```python
from build123d import *

# Parameters (mm, degrees)
SKETCH1_R           = 6.9
BOSS_EXTRUDE1_DEPTH = 24.8
SKETCH2_R           = 1.9
CUT_EXTRUDE1_DEPTH  = 24.8
SKETCH3_R           = 4
CUT_EXTRUDE2_DEPTH  = 10
SKETCH4_R           = 2
CUT_EXTRUDE3_DEPTH  = 10


with BuildPart() as part:
    # Sketch1 → Boss-Extrude1 (new body)
    with BuildSketch(Plane.XY):
        with Locations(Location((0.333575811, 0, 0), (0, 0, 180))):
            Circle(SKETCH1_R)
    extrude(amount=BOSS_EXTRUDE1_DEPTH)

    # Sketch2 → Cut-Extrude1 (cut)
    with BuildSketch(Plane(origin=(0, 6.9, 0), x_dir=(1, 0, 0), z_dir=(0, 1, 0))):
        with Locations(Location((0.515412316, -4, 0), (0, 0, 270))):
            Circle(SKETCH2_R)
        with Locations(Location((0.515412316, -20.8, 0), (0, 0, 270))):
            Circle(SKETCH2_R)
    extrude(amount=-CUT_EXTRUDE1_DEPTH, mode=Mode.SUBTRACT)

    # Sketch3 → Cut-Extrude2 (cut)
    with BuildSketch(Plane.XY.offset(24.8)):
        Circle(SKETCH3_R)
    extrude(amount=-CUT_EXTRUDE2_DEPTH, mode=Mode.SUBTRACT)

    # Sketch4 → Cut-Extrude3 (cut)
    with BuildSketch(Plane(origin=(0, 0, 0), x_dir=(-1, 0, 0), z_dir=(0, 0, -1))):
        Circle(SKETCH4_R)
    extrude(amount=-CUT_EXTRUDE3_DEPTH, mode=Mode.SUBTRACT)


solid = part.part
```
Design review of the part built by this model. Coordinates are the model's own, in mm. A direction names the side the tool comes from. Give positions to 0.01 mm unless a question says otherwise; leave off trailing zeros. Write each loop counter-clockwise with the first axis right and the second up, starting at its lowest first coordinate (ties: lowest second). Pieces come first, ordered by that corner, then holes. Notation, with made-up numbers: (65.5, -25) -> (86.5, -25) arc R19 cw to (86.5, -9) -> close; hole circle Ø5 at (-6.75, 28.5). An arc over 180 degrees is marked (long way). Answer in a Markdown table with one row per item.
(1) Consider section B-B (y = 6). State the section outline as (x, z) points, then the cut area to 3 significant figures.
Results:
| item | result |
|---|---|
| outline | (-3.07, 0) -> (3.74, 0) -> (3.74, 24.8) -> (-3.07, 24.8) -> close; hole circle Ø3.8 at (0.52, 4); hole circle Ø3.8 at (0.52, 20.8) |
| area | 146 mm2 |
(2) Consider section A-A (z = 4). State the section outline as (x, y) points.
Results:
| item | result |
|---|---|
| outline | (-1.38, -6.68) -> (-1.38, -1.44) arc R2 cw to (-1.38, 1.44) -> (-1.38, 6.68) arc R6.9 ccw to start; (2.42, -6.58) arc R6.9 ccw to (2.42, 6.58) -> close |
(3) To check wall thickness, follow probe 1 along Z at (x, y) = (-0.75, -1.5); probe 2 along Z at (x, y) = (-1.5, 2.5); probe 3 along Y at (x, z) = (0, 6.5). State the ranges of each line that lie inside material, in increasing order.
Results:
| item | result |
|---|---|
| probe 1 | 10 to 14.8 |
| probe 2 | 0 to 14.8 |
| probe 3 | -6.89 to -2, 2 to 6.89 |
(4) Clearance check with flat-ended pins moving along their axes: pin 1 (5 mm diameter, centred on y = -0.5, z = 7, fed in from -X); pin 2 (6.5 mm diameter, centred on x = 0, y = 0.5, fed in from +Z); pin 3 (3 mm diameter, centred on x = 0.52, z = 20.8, fed in from +Y); pin 4 (2 mm diameter, centred on y = -4, z = 11, fed in from -X). State where each tip first meets the part, or that it passes through.
Results:
| item | result |
|---|---|
| pin 1 | x = -6.57 |
| pin 2 | z = 14.8 |
| pin 3 | through |
| pin 4 | x = -5.88 |
(5) Consider section D-D (y = 0). State the section outline as (x, z) points.
Results:
| item | result |
|---|---|
| outline | (-6.57, 0) -> (-2, 0) -> (-2, 10) -> (2, 10) -> (2, 5.19) arc R1.9 cw to (2, 2.81) -> (2, 0) -> (7.23, 0) -> (7.23, 24.8) -> (4, 24.8) -> (4, 14.8) -> (-4, 14.8) -> (-4, 24.8) -> (-6.57, 24.8) -> close |
(6) Consider section C-C (x = 0). State the section outline as (y, z) points, then the cut area to 3 significant figures.
Results:
| item | result |
|---|---|
| outline | (-6.89, 0) -> (-2, 0) -> (-2, 2.17) -> (-6.89, 2.17) -> close; (-6.89, 5.83) -> (-2, 5.83) -> (-2, 10) -> (2, 10) -> (2, 5.83) -> (6.89, 5.83) -> (6.89, 18.97) -> (4, 18.97) -> (4, 14.8) -> (-4, 14.8) -> (-4, 18.97) -> (-6.89, 18.97) -> close; (-6.89, 22.63) -> (-4, 22.63) -> (-4, 24.8) -> (-6.89, 24.8) -> close; (2, 0) -> (6.89, 0) -> (6.89, 2.17) -> (2, 2.17) -> close; (4, 22.63) -> (6.89, 22.63) -> (6.89, 24.8) -> (4, 24.8) -> close |
| area | 165 mm2 |
(7) Mouldability with a two-part tool opening along X and no side actions: class faces 1 (the cylindrical face through (-2.95, 2.7, 19.87)), 2 (the flat face through (-3, -3, 24.8)), 3 (the cylindrical face through (-6.25, -2.07, 12.23)) as +X half, -X half, draft (parallel to the pull), parting line (faces both ways), or undercut.
Results:
| item | result |
|---|---|
| face 1 | undercut |
| face 2 | draft |
| face 3 | parting line |
(8) For faces 4 (the flat face through (0, 0, 10)), 5 (the flat face through (0, 0, 14.8)), 6 (the cylindrical face through (2.4, 5.07, 20.55)), list the 3-axis set-ups (+Z, -Z, +X, -X, +Y, -Y) from which the entire face can be reached by the end or side of a thin tool; tool diameter is ignored.
Results:
| item | result |
|---|---|
| face 4 | -Z |
| face 5 | +Z |
| face 6 | +Y, -Y |
